Build history of the part. All positions in model axes, mm. Face numbers are marked on the shaded views. A direction names the side the tool comes from. Coordinates: 2 decimals unless noted, no trailing zeros. Loops run counter-clockwise (first coordinate to the right, second up) from the corner with the lowest first, then second, coordinate; pieces in that order, holes last. Notation, with made-up numbers: M 51,61 L 69,61 A20 ccw 69,73 Z; hole C -17.5,-12.75 d3. An arc over 180 degrees is marked long. Write each question's results on one line, items separated by ' | '. Start each with the question number.
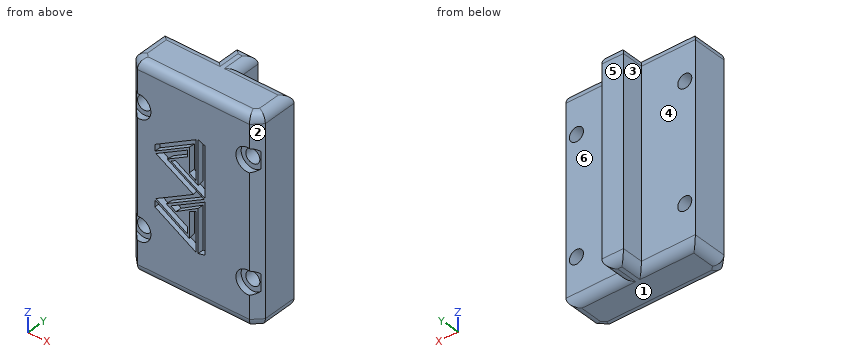
from build123d import *

# Parameters (mm, degrees)
SKETCH1_W                    = 30
SKETCH1_H                    = 47
BOSS_EXTRUDE1_DEPTH          = 10
SKETCH2_W                    = 5
SKETCH2_H                    = 47
BOSS_EXTRUDE2_DEPTH          = 5
SKETCH3_R                    = 1.625
CUT_EXTRUDE1_DEPTH           = 32.658332237
SKETCH4_R                    = 2.7
CUT_EXTRUDE2_DEPTH           = 1.45
CHAMFER1_SIZE                = 2
CHAMFER2_SIZE                = 2
FILLET1_R                    = 2
FILLET2_R                    = 2
CUT_EXTRUDE6_DEPTH           = 1.5
CUT_EXTRUDE6_DRAFT           = 4
CUT_EXTRUDE6_PROFILE_2_DEPTH = 1.5
CUT_EXTRUDE6_PROFILE_2_DRAFT = 4
CUT_EXTRUDE6_PROFILE_3_DEPTH = 1.5
CUT_EXTRUDE6_PROFILE_3_DRAFT = 4
CUT_EXTRUDE6_PROFILE_4_DEPTH = 1.5
CUT_EXTRUDE6_PROFILE_4_DRAFT = 4
CUT_EXTRUDE6_PROFILE_5_DEPTH = 1.5
CUT_EXTRUDE6_PROFILE_5_DRAFT = 4


with BuildPart() as part:
    # Sketch1 → Boss-Extrude1 (new body)
    with BuildSketch(Plane(origin=(0, 0, 0), x_dir=(1, 0, 0), z_dir=(0, 1, 0))):
        Rectangle(SKETCH1_W, SKETCH1_H)
    extrude(amount=BOSS_EXTRUDE1_DEPTH)

    # Sketch2 → Boss-Extrude2 (add)
    with BuildSketch(Plane(origin=(0, 10, 0), x_dir=(1, 0, 0), z_dir=(0, 1, 0))):
        Rectangle(SKETCH2_W, SKETCH2_H)
    extrude(amount=BOSS_EXTRUDE2_DEPTH)

    # Sketch3 → Cut-Extrude1 (cut, through all)
    with BuildSketch(Plane.XZ):
        with Locations(Location((-12.56, 13.5, 0), (0, 0, 270))):
            Circle(SKETCH3_R)
        with Locations(Location((-12.56, -13.5, 0), (0, 0, 270))):
            Circle(SKETCH3_R)
        with Locations(Location((12.56, -13.5, 0), (0, 0, 270))):
            Circle(SKETCH3_R)
        with Locations(Location((12.56, 13.5, 0), (0, 0, 270))):
            Circle(SKETCH3_R)
    extrude(amount=-CUT_EXTRUDE1_DEPTH, mode=Mode.SUBTRACT)

    # Sketch4 → Cut-Extrude2 (cut)
    with BuildSketch(Plane.XZ):
        with Locations((-12.56, 13.5)):
            Circle(SKETCH4_R)
        with Locations((-12.56, -13.5)):
            Circle(SKETCH4_R)
        with Locations((12.56, -13.5)):
            Circle(SKETCH4_R)
        with Locations((12.56, 13.5)):
            Circle(SKETCH4_R)
    extrude(amount=-CUT_EXTRUDE2_DEPTH, mode=Mode.SUBTRACT)

    # Chamfer1
    # the kernel refuses this chamfer: 2 mm, written as the material it takes off along each edge
    with BuildSketch(Plane(origin=(-15, 0, -28.643365976), x_dir=(0.9996219169112968, -0.027495876610586365, 0), z_dir=(0, 0, 1)), Plane(origin=(-15, 0, 9.512661705), x_dir=(0.9996219169112968, -0.027495876610586365, 0), z_dir=(0, 0, 1))) as chamfer1_piece_1:
        Polygon((CHAMFER1_SIZE * 0.999621916911, CHAMFER1_SIZE * 0.0274958766106), (-CHAMFER1_SIZE * 0.0274958766106, CHAMFER1_SIZE * 0.999621916911), (0, 0), align=None)
    extrude(amount=19.130704271, mode=Mode.SUBTRACT)
    with BuildSketch(Plane(origin=(-15, 0, -17.487338295), x_dir=(0.9996219169112968, -0.027495876610586365, 0), z_dir=(0, 0, 1))) as chamfer1_piece_2:
        Polygon((CHAMFER1_SIZE * 0.999621916911, CHAMFER1_SIZE * 0.0274958766106), (-CHAMFER1_SIZE * 0.0274958766106, CHAMFER1_SIZE * 0.999621916911), (0, 0), align=None)
    extrude(amount=34.974676589, mode=Mode.SUBTRACT)

    # Chamfer2
    # the kernel refuses this chamfer: 2 mm, written as the material it takes off along each edge
    with BuildSketch(Plane(origin=(15, 0, 28.643365976), x_dir=(0.027495876610586494, 0.9996219169112968, 0), z_dir=(0, 0, -1)), Plane(origin=(15, 0, -9.512661705), x_dir=(0.027495876610586494, 0.9996219169112968, 0), z_dir=(0, 0, -1))) as chamfer2_piece_1:
        Polygon((CHAMFER2_SIZE * 0.999621916911, -CHAMFER2_SIZE * 0.0274958766106), (-CHAMFER2_SIZE * 0.0274958766106, -CHAMFER2_SIZE * 0.999621916911), (0, 0), align=None)
    extrude(amount=19.130704271, mode=Mode.SUBTRACT)
    with BuildSketch(Plane(origin=(15, 0, 17.487338295), x_dir=(0.027495876610586494, 0.9996219169112968, 0), z_dir=(0, 0, -1))) as chamfer2_piece_2:
        Polygon((CHAMFER2_SIZE * 0.999621916911, -CHAMFER2_SIZE * 0.0274958766106), (-CHAMFER2_SIZE * 0.0274958766106, -CHAMFER2_SIZE * 0.999621916911), (0, 0), align=None)
    extrude(amount=34.974676589, mode=Mode.SUBTRACT)

    # Fillet1
    fillet1_edges = [part.edges().sort_by_distance(p)[0] for p in [
        (-14, 1, 23.5),
        (-15, 6, 23.5),
        (-8.75, 10, 23.5),
        (-2.5, 12.5, 23.5),
        (0, 15, 23.5),
        (2.5, 12.5, 23.5),
        (8.75, 10, 23.5),
        (15, 6, 23.5),
        (14, 1, 23.5),
        (0, 0, 23.5),
    ]]
    fillet(fillet1_edges, radius=FILLET1_R)

    # Fillet2
    fillet2_edges = [part.edges().sort_by_distance(p)[0] for p in [
        (8.75, 10, -23.5),
        (2.5, 12.5, -23.5),
        (0, 15, -23.5),
        (-2.5, 12.5, -23.5),
        (-8.75, 10, -23.5),
        (-15, 6, -23.5),
        (-14, 1, -23.5),
        (0, 0, -23.5),
        (14, 1, -23.5),
        (15, 6, -23.5),
    ]]
    fillet(fillet2_edges, radius=FILLET2_R)


with BuildPart() as cut_extrude6_tool:
    # Mobious Logo → Cut-Extrude6 (with draft: the straight prism first)
    with BuildSketch(Plane.XZ):
        Polygon((-8.928580544, -5.393458037), (-8.928580544, -6.93818631), (0.653971114, -12.514917192), (0.653971114, -3.429820402), (-0.949401841, -4.248746813), (-0.949401841, -10.158552031), align=None)
    extrude(amount=-CUT_EXTRUDE6_DEPTH)
    # Cut-Extrude6: the draft: its side faces are tilted about the plane it starts from
    cut_extrude6_sides = [cut_extrude6_tool.faces().sort_by_distance(p)[0] for p in [
        (-8.928580544, 0.75, -6.165822173),
        (-4.137304715, 0.75, -9.726551751),
        (0.653971114, 0.75, -7.972368797),
        (-0.147715364, 0.75, -3.839283608),
        (-0.949401841, 0.75, -7.203649422),
        (-4.938991193, 0.75, -7.776005034),
    ]]
    draft(cut_extrude6_sides, Plane.XZ, CUT_EXTRUDE6_DRAFT)


with BuildPart() as part_1:
    add(part.part)

    # Cut-Extrude6: cut by cut_extrude6_tool
    add(cut_extrude6_tool.part, mode=Mode.SUBTRACT)


with BuildPart() as cut_extrude6_profile_2_tool:
    # Mobious Logo → Cut-Extrude6 profile 2 (with draft: the straight prism first)
    with BuildSketch(Plane.XZ):
        Polygon((-4.084941045, -5.681458223), (1.099062311, -2.555426049), (1.099062311, -12.520785535), (2.643790584, -12.174553336), (2.643790584, -0.471273032), (-5.23694179, -4.974548675), align=None)
    extrude(amount=-CUT_EXTRUDE6_PROFILE_2_DEPTH)
    # Cut-Extrude6 profile 2: the draft: its side faces are tilted about the plane it starts from
    cut_extrude6_profile_2_sides = [cut_extrude6_profile_2_tool.faces().sort_by_distance(p)[0] for p in [
        (-1.492939367, 0.75, -4.118442136),
        (1.099062311, 0.75, -7.538105792),
        (1.871426448, 0.75, -12.347669435),
        (2.643790584, 0.75, -6.322913184),
        (-1.296575603, 0.75, -2.722910854),
        (-4.660941418, 0.75, -5.328003449),
    ]]
    draft(cut_extrude6_profile_2_sides, Plane.XZ, CUT_EXTRUDE6_PROFILE_2_DRAFT)


with BuildPart() as part_2:
    add(part_1.part)

    # Cut-Extrude6 profile 2: cut by cut_extrude6_profile_2_tool
    add(cut_extrude6_profile_2_tool.part, mode=Mode.SUBTRACT)


with BuildPart() as cut_extrude6_profile_3_tool:
    # Mobious Logo → Cut-Extrude6 profile 3 (with draft: the straight prism first)
    with BuildSketch(Plane.XZ):
        Polygon((-1.414393861, -9.346915142), (-1.414393861, -7.767367916), (-6.320622953, -4.974548675), (2.486400923, 0.065282344), (-6.091859658, 4.94836684), (-1.414393861, 7.625052806), (-1.414393861, 9.113526764), (-8.692944028, 4.94836684), (0, 0), (-8.692944028, -4.974548675), align=None)
    extrude(amount=-CUT_EXTRUDE6_PROFILE_3_DEPTH)
    # Cut-Extrude6 profile 3: the draft: its side faces are tilted about the plane it starts from
    cut_extrude6_profile_3_sides = [cut_extrude6_profile_3_tool.faces().sort_by_distance(p)[0] for p in [
        (-1.414393861, 0.75, -8.557141529),
        (-3.867508407, 0.75, -6.370958296),
        (-1.917111015, 0.75, -2.454633165),
        (-1.802729367, 0.75, 2.506824592),
        (-3.75312676, 0.75, 6.286709823),
        (-1.414393861, 0.75, 8.369289785),
        (-5.053668945, 0.75, 7.030946802),
        (-4.346472014, 0.75, 2.47418342),
        (-4.346472014, 0.75, -2.487274337),
        (-5.053668945, 0.75, -7.160731908),
    ]]
    draft(cut_extrude6_profile_3_sides, Plane.XZ, CUT_EXTRUDE6_PROFILE_3_DRAFT)


with BuildPart() as part_3:
    add(part_2.part)

    # Cut-Extrude6 profile 3: cut by cut_extrude6_profile_3_tool
    add(cut_extrude6_profile_3_tool.part, mode=Mode.SUBTRACT)


with BuildPart() as cut_extrude6_profile_4_tool:
    # Mobious Logo → Cut-Extrude6 profile 4 (with draft: the straight prism first)
    with BuildSketch(Plane.XZ):
        Polygon((-8.928580544, 5.393458037), (-0.949401841, 9.975279185), (-0.949401841, 4.293820961), (0.653971114, 3.272729391), (0.653971114, 12.384008017), (-8.928580544, 6.859640804), align=None)
    extrude(amount=-CUT_EXTRUDE6_PROFILE_4_DEPTH)
    # Cut-Extrude6 profile 4: the draft: its side faces are tilted about the plane it starts from
    cut_extrude6_profile_4_sides = [cut_extrude6_profile_4_tool.faces().sort_by_distance(p)[0] for p in [
        (-4.938991193, 0.75, 7.684368611),
        (-0.949401841, 0.75, 7.134550073),
        (-0.147715364, 0.75, 3.783275176),
        (0.653971114, 0.75, 7.828368704),
        (-4.137304715, 0.75, 9.62182441),
        (-8.928580544, 0.75, 6.126549421),
    ]]
    draft(cut_extrude6_profile_4_sides, Plane.XZ, CUT_EXTRUDE6_PROFILE_4_DRAFT)


with BuildPart() as part_4:
    add(part_3.part)

    # Cut-Extrude6 profile 4: cut by cut_extrude6_profile_4_tool
    add(cut_extrude6_profile_4_tool.part, mode=Mode.SUBTRACT)


with BuildPart() as cut_extrude6_profile_5_tool:
    # Mobious Logo → Cut-Extrude6 profile 5 (with draft: the straight prism first)
    with BuildSketch(Plane.XZ):
        Polygon((-5.23694179, 4.94836684), (2.643790584, 0.418909362), (2.643790584, 11.965098655), (1.099062311, 12.577663315), (1.099062311, 2.487274337), (-4.143752967, 5.500586773), align=None)
    extrude(amount=-CUT_EXTRUDE6_PROFILE_5_DEPTH)
    # Cut-Extrude6 profile 5: the draft: its side faces are tilted about the plane it starts from
    cut_extrude6_profile_5_sides = [cut_extrude6_profile_5_tool.faces().sort_by_distance(p)[0] for p in [
        (-1.296575603, 0.75, 2.683638101),
        (2.643790584, 0.75, 6.192004008),
        (1.871426448, 0.75, 12.271380985),
        (1.099062311, 0.75, 7.532468826),
        (-1.522345328, 0.75, 3.993930555),
        (-4.690347379, 0.75, 5.224476806),
    ]]
    draft(cut_extrude6_profile_5_sides, Plane.XZ, CUT_EXTRUDE6_PROFILE_5_DRAFT)


with BuildPart() as part_5:
    add(part_4.part)

    # Cut-Extrude6 profile 5: cut by cut_extrude6_profile_5_tool
    add(cut_extrude6_profile_5_tool.part, mode=Mode.SUBTRACT)


solid = part_5.part
1. Wall check: line 1 along X through (y, z) = (4, -13.5) (3 decimals); line 2 along Z through (x, y) = (-13, 6.5); line 3 along X through (y, z) = (1.25, -5). Give the ranges that are in metal, low to high.
2. Band-saw the part on B-B, the plane y = 10.5. List the corners of the cut face in (x, z), plus the area to 3 significant figures.
3. Mould opens along X. For the marked faces 1, 2 and 3 say: +X half, -X half, draft (parallel to the pull), parting line (faces both ways), or undercut.
4. Which spindle directions (+Z, -Z, +X, -X, +Y, -Y) get a long thin tool onto all of the face, cutting with end or side? Do the marked faces 4, 5 and 6. Say none if no direction does.
5. Band-saw the part on D-D, the plane z = -14. List the corners of the cut face in (x, y).
6. Band-saw the part on C-C, the plane y = 3.5. List the corners of the cut face in (x, z) (3 decimals).
7. Pin check, flat tips, straight feed: pin 1 (3 mm diameter, centred on x = -3.5, z = 7, fed in from -Y); pin 2 (10 mm diameter, centred on x = -8.5, z = 0.5, fed in from +Y); pin 3 (3.5 mm diameter, centred on x = -12.56, z = 13.5, fed in from -Y). Stop position of each tip, or through.
8. Band-saw the part on A-A, the plane z = 13.5. List the corners of the cut face in (x, y) (3 decimals), plus the area to 3 significant figures.
Checked values:
1) line 1: -15 to -14.185, -10.935 to 10.935, 14.185 to 15 | line 2: -23.5 to -15.06, -11.94 to 11.94, 15.06 to 23.5 | line 3: -14.25 to -8.82, -6.1 to -5.36, -2.79 to -1.04, 0.74 to 1.01, 2.73 to 14.25
2) outline: M -2.5,-21.5 A2 ccw -0.5,-23.5 L 0.5,-23.5 A2 ccw 2.5,-21.5 L 2.5,21.5 A2 ccw 0.5,23.5 L -0.5,23.5 A2 ccw -2.5,21.5 Z | area: 232 mm²
3) face 1: draft | face 2: +X half | face 3: -X half
4) face 4: +Z, -Z, -X, +Y | face 5: +Z, -Z, +X, -X, +Y | face 6: +Z, -Z, +X, +Y
5) outline: M -15,2 L -14.45,1.45 L -14.11,1.45 L -14.11,10 L -15,10 Z; M -11.01,1.45 L -9.91,1.45 L -9.91,0 L 9.91,0 L 9.91,1.45 L 11.01,1.45 L 11.01,10 L 2.5,10 L 2.5,15 L -2.5,15 L -2.5,10 L -11.01,10 Z; M 14.11,1.45 L 14.45,1.45 L 15,2 L 15,10 L 14.11,10 Z
6) outline: M -15,-21.5 A2 ccw -13,-23.5 L 13,-23.5 A2 ccw 15,-21.5 L 15,21.5 A2 ccw 13,23.5 L -13,23.5 A2 ccw -15,21.5 Z; hole C -12.56,-13.5 d3.25; hole C -12.56,13.5 d3.25; hole C 12.56,-13.5 d3.25; hole C 12.56,13.5 d3.25
7) pin 1: y = 0 | pin 2: y = 10 | pin 3: y = 1.45
8) outline: M -15,2 L -14.45,1.45 L -14.185,1.45 L -14.185,10 L -15,10 Z; M -10.935,1.45 L -9.86,1.45 L -9.86,0 L 9.86,0 L 9.86,1.45 L 10.935,1.45 L 10.935,10 L 2.5,10 L 2.5,15 L -2.5,15 L -2.5,10 L -10.935,10 Z; M 14.185,1.45 L 14.45,1.45 L 15,2 L 15,10 L 14.185,10 Z | area: 254 mm²
